Check sheet for the modelled part. Datum: model origin and axes. Units: mm. Face numbers are marked on the shaded views. Give positions to 0.01 mm unless a question says otherwise; leave off trailing zeros. Write each loop counter-clockwise with the first axis right and the second up, starting at its lowest first coordinate (ties: lowest second). Pieces come first, ordered by that corner, then holes. Notation, with made-up numbers: M -37.5,81.25 L -1.5,81.25 A27 ccw -1.5,100.25 Z; hole C 82.5,16 d11. An arc over 180 degrees is marked long. Write item = value, one per line. Start each with the question number.
1) Sectioned sample at D-D, the plane y = 20. Record the cut outline in (x, z).
2) Scan lines: L1, parallel to Y at x = 0, z = 2.8 (3 decimals); L2, parallel to X at y = -0.5, z = 8.75; L3, parallel to X at y = 7, z = 3.75. Record each from-to range of solid material in increasing order.
3) Sectioned sample at C-C, the plane z = 7.5. Record the cut outline in (x, y).
4) Sectioned sample at A-A, the plane y = 0. Record the cut outline in (x, z) (3 decimals), then the cut area to 3 significant figures.
5) Sectioned sample at B-B, the plane x = 0. Record the cut outline in (y, z) (3 decimals), then the cut area to 3 significant figures.
6) Draft check along X on the marked faces 1, 2 and 3. Enter one of: pulls with the +X half, pulls with the -X half, needs draft (parallel to the pull), parting line crosses it, or undercut.
7) Gauge pin test, flat ends, axial feed: pin 1 (4 mm diameter, centred on y = -11, z = 1.5, fed in from +X); pin 2 (5 mm diameter, centred on x = 8.5, z = 1.5, fed in from -Y); pin 3 (1.5 mm diameter, centred on x = -15.5, z = 6.5, fed in from +Y). Record the tip position at first contact, or that the pin passes through.
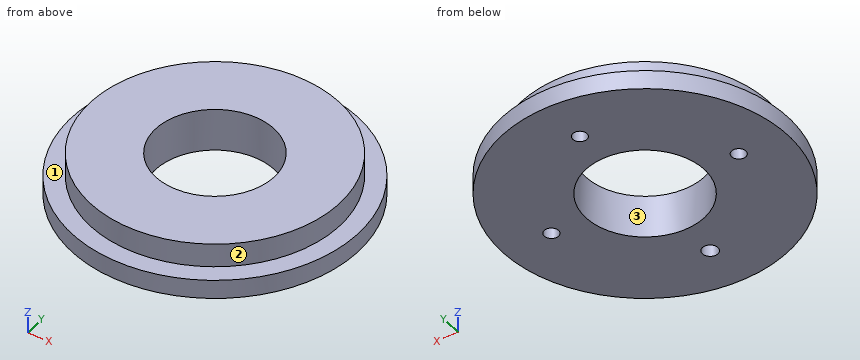
from build123d import *

# Parameters (mm, degrees)
SKETCH2_R             = 30.165
SKETCH2_R_2           = 12.5
BOSS_EXTRUDE1_DEPTH   = 4
SKETCH3_R             = 26.25
SKETCH3_R_2           = 12.5
BOSS_EXTRUDE2_DEPTH   = 5
CROQUIS1_R            = 1.5
CROQUIS1_R_2          = 1.636681132
CORTAR_EXTRUIR1_DEPTH = 5


with BuildPart() as part:
    # Sketch2 → Boss-Extrude1 (new body)
    with BuildSketch(Plane.XY):
        Circle(SKETCH2_R)
        Circle(SKETCH2_R_2, mode=Mode.SUBTRACT)
    extrude(amount=BOSS_EXTRUDE1_DEPTH)

    # Sketch3 → Boss-Extrude2 (add)
    with BuildSketch(Plane.XY.offset(4)):
        Circle(SKETCH3_R)
        Circle(SKETCH3_R_2, mode=Mode.SUBTRACT)
    extrude(amount=BOSS_EXTRUDE2_DEPTH)

    # Croquis1 → Cortar-Extruir1 (cut)
    with BuildSketch(Plane(origin=(0, 0, 0), x_dir=(-1, 0, 0), z_dir=(0, 0, -1))):
        with Locations((0, 20)):
            Circle(CROQUIS1_R)
        with Locations((0, -20)):
            Circle(CROQUIS1_R_2)
        with Locations((20, 0)):
            Circle(CROQUIS1_R)
        with Locations((-20, 0)):
            Circle(CROQUIS1_R)
    extrude(amount=-CORTAR_EXTRUIR1_DEPTH, mode=Mode.SUBTRACT)


solid = part.part
Data:
q1.outline = M -22.58,0 L -1.5,0 L -1.5,5 L 1.5,5 L 1.5,0 L 22.58,0 L 22.58,4 L 17,4 L 17,9 L -17,9 L -17,4 L -22.58,4 Z
q2.L1 = -30.165 to -21.637, -18.363 to -12.5, 12.5 to 18.5, 21.5 to 30.165
q2.L2 = -26.25 to -12.49, 12.49 to 26.25
q2.L3 = -29.34 to -10.36, 10.36 to 29.34
q3.outline = C 0,0 d52.5; hole C 0,0 d25
q4.outline = M -30.165,0 L -21.5,0 L -21.5,5 L -18.5,5 L -18.5,0 L -12.5,0 L -12.5,9 L -26.25,9 L -26.25,4 L -30.165,4 Z; M 12.5,0 L 18.5,0 L 18.5,5 L 21.5,5 L 21.5,0 L 30.165,0 L 30.165,4 L 26.25,4 L 26.25,9 L 12.5,9 Z
q4.area = 249 mm2
q5.outline = M -30.165,0 L -21.637,0 L -21.637,5 L -18.363,5 L -18.363,0 L -12.5,0 L -12.5,9 L -26.25,9 L -26.25,4 L -30.165,4 Z; M 12.5,0 L 18.5,0 L 18.5,5 L 21.5,5 L 21.5,0 L 30.165,0 L 30.165,4 L 26.25,4 L 26.25,9 L 12.5,9 Z
q5.area = 247 mm2
q6.face_1 = needs draft
q6.face_2 = parting line crosses it
q6.face_3 = undercut
q7.pin_1 = 28.79
q7.pin_2 = -29.56
q7.pin_3 = 21.71
